Drawing for the job (mm, zero at the part's lowest x, y, z). A direction names the side the tool comes from. Give positions to 0.01 mm unless a question says otherwise; leave off trailing zeros. Write each loop counter-clockwise with the first axis right and the second up, starting at its lowest first coordinate (ties: lowest second). Pieces come first, ordered by that corner, then holes.
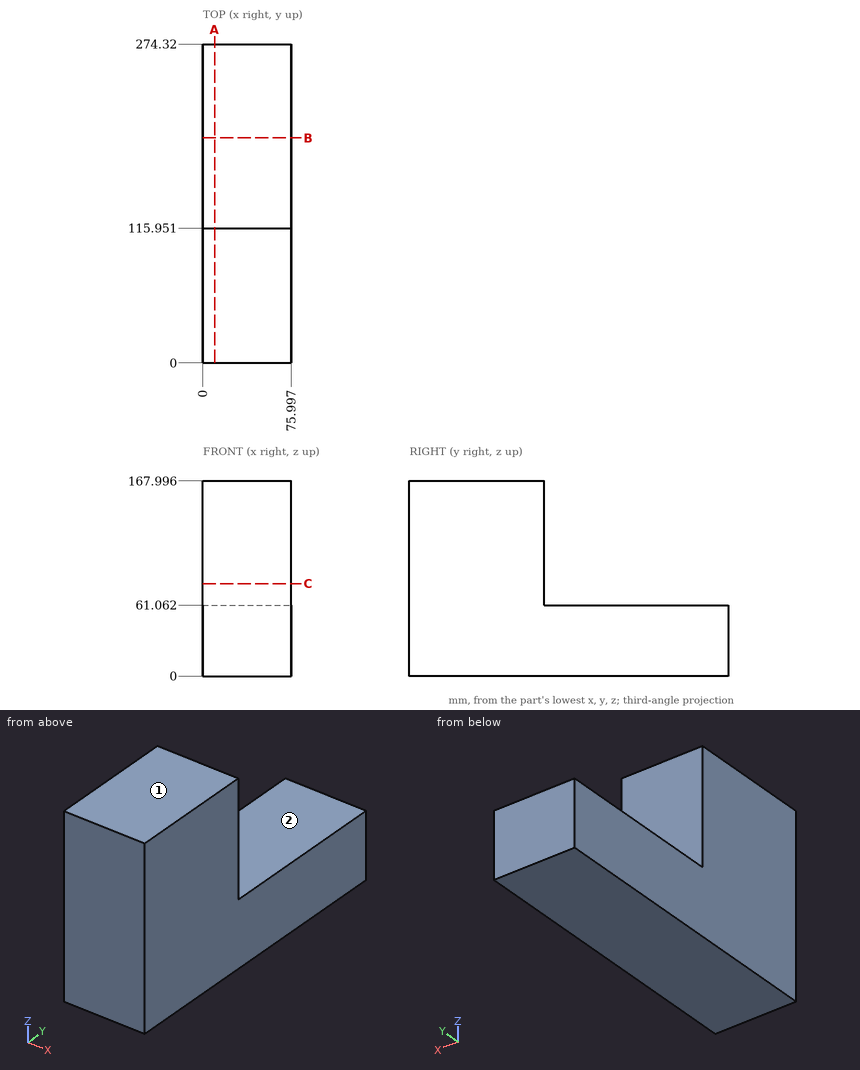
1. Pin check, flat tips, straight feed: P1, Ø1, axis at x = 44, z = 146, coming from the +Y side; P2, Ø1, axis at x = 9.5, y = 171.5, coming from the +Z side. Stop position of each tip, or through.
Calculated:
P1: stops at y = 115.95
P2: stops at z = 61.06
2. Probe probe 1 along Z at (x, y) = (7.5, 253); probe 2 along Y at (x, z) = (71, 117). List the from-to ranges inside material, lowest first.
Calculated:
probe 1: z = 0 to 61.06
probe 2: y = 0 to 115.95
3. Slice it at B-B, the plane y = 193.5. Write the cut outline in (x, z), and give its area (3 significant figures).
Calculated:
outline: (0, 0) - (76, 0) - (76, 61.06) - (0, 61.06) - close
area: 4,640 mm2
4. Slice it at C-C, the plane z = 79.5. Write the cut outline in (x, y).
Calculated:
outline: (0, 0) - (76, 0) - (76, 115.95) - (0, 115.95) - close
5. Slice it at A-A, the plane x = 10. Write the cut outline in (y, z) (1 decimal), and give its area (4 significant figures).
Calculated:
outline: (0, 0) - (274.3, 0) - (274.3, 61.1) - (116, 61.1) - (116, 168) - (0, 168) - close
area: 29,150 mm2
6. Which spindle directions (+Z, -Z, +X, -X, +Y, -Y) get a long thin tool onto all of the face, cutting with end or side? Do the marked faces 1 and 2. Say none if no direction does.
Calculated:
face 1: +Z, +X, -X, +Y, -Y
face 2: +Z, +X, -X, +Y
